Study the drawing (mm; zero at the part's minimum x, y, z) and answer. Give positions to 0.01 mm unless a question says otherwise; leave off trailing zeros. Answer as CSV lines item,"result".
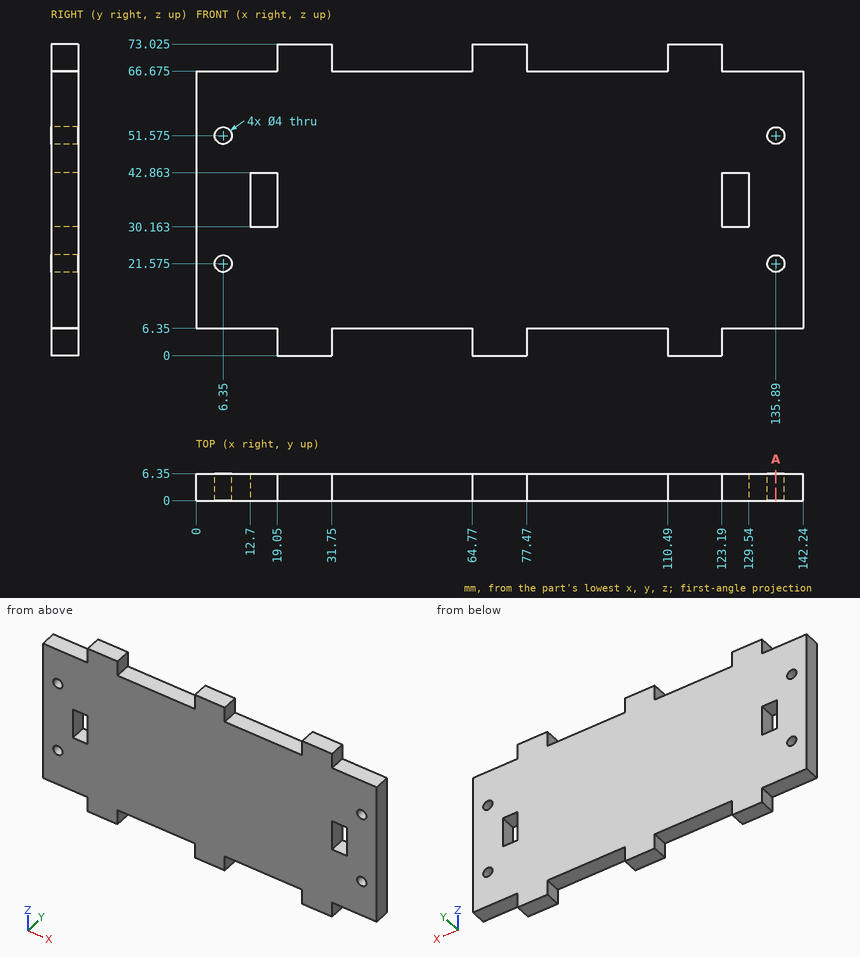
(1) Find the intervals of material crossed by L1, parallel to X at y = 6.25, z = 36.5; L2, parallel to X at y = 6, z = 22 (1 decimal), in increasing order.
Worked out:
L1,"x = 0 to 12.7, 19.05 to 123.19, 129.54 to 142.24"
L2,"x = 0 to 4.4, 8.3 to 133.9, 137.8 to 142.2"
(2) A cutting plane is placed at A-A (x = 135.89). Count the separate pieces of the cut face and the enclosed holes in it, and give its area (3 significant figures).
Worked out:
separate pieces,"3"
enclosed holes,"0"
area,"332 mm^2"
(3) Each of these flat-tipped pins is pushed along its axis until it touches: P1, Ø1.9, axis at y = 2, z = 70.5, coming from the +X side; P2, Ø1.9, axis at x = 48, y = 3.5, coming from the -Z side. Where does it stop, or does it pass through?
Worked out:
P1,"stops at x = 123.19"
P2,"stops at z = 6.35"
